```python
from build123d import *

# Parameters (mm, degrees)
BOSS_EXTRUDE1_DEPTH             = 3
CUT_EXTRUDE1_DEPTH              = 19.761966848
SKETCH3_W                       = 16.06
SKETCH3_H                       = 1.22
CUT_EXTRUDE2_DEPTH              = 3
CUT_EXTRUDE3_DEPTH              = 12.557681428
CUT_EXTRUDE3_DEPTH_BACK         = 12.557681428
SKETCH5_W                       = 1.3
SKETCH5_H                       = 3.6
CUT_EXTRUDE4_DEPTH              = 1.6
CUT_EXTRUDE5_DEPTH              = 1.6
SKETCH8_W                       = 0.3
SKETCH8_H                       = 1.3
BOSS_EXTRUDE3_DEPTH             = 0.3
CUT_EXTRUDE6_REACH              = 13.558
SKETCH9_W                       = 0.97
SKETCH9_H                       = 0.7
SKETCH10_W                      = 1.3
SKETCH10_H                      = 0.995055469
CUT_EXTRUDE7_DEPTH              = 0.3
SKETCH11_W                      = 1.3
SKETCH11_H                      = 1.339878891
CUT_EXTRUDE8_DEPTH              = 0.3
SKETCH12_W                      = 0.22
SKETCH12_H                      = 2.3
BOSS_EXTRUDE4_DEPTH             = 0.3
SZKIC1_W                        = 4.81
SZKIC1_H                        = 6.619114068
WYTNIJ_WYCI_GNI_CIE1_DEPTH      = 12.050452479
WYTNIJ_WYCI_GNI_CIE1_DEPTH_BACK = 12.050452479


with BuildPart() as part:
    # Sketch1 → Boss-Extrude1 (new body)
    with BuildSketch(Plane.XY):
        with BuildLine():
            Line((4.729085478, -2.65), (4.875, -2.504085478))
            Line((4.875, -2.504085478), (5.125, -2.504085478))
            Line((5.125, -2.504085478), (5.270914522, -2.65))
            Line((5.270914522, -2.65), (5.729085478, -2.65))
            Line((5.729085478, -2.65), (5.875, -2.504085478))
            Line((5.875, -2.504085478), (6.125, -2.504085478))
            Line((6.125, -2.504085478), (6.270914522, -2.65))
            Line((6.270914522, -2.65), (6.729085478, -2.65))
            Line((6.729085478, -2.65), (6.875, -2.504085478))
            Line((6.875, -2.504085478), (7.125, -2.504085478))
            Line((7.125, -2.504085478), (7.270914522, -2.65))
            Line((7.270914522, -2.65), (10.3, -2.65))
            Line((10.3, -2.65), (10.3, 1.65))
            Line((10.3, 1.65), (9.52, 1.65))
            Line((9.52, 1.65), (9.52, -1.49))
            ThreePointArc((9.52, -1.49), (9.26, -1.75), (9, -1.49))
            Line((9, -1.49), (9, 1.65))
            Line((9, 1.65), (8.03, 1.65))
            Line((8.03, 1.65), (8.03, 2.65))
            Line((8.03, 2.65), (-8.03, 2.65))
            Line((-8.03, 2.65), (-8.03, 1.65))
            Line((-8.03, 1.65), (-9, 1.65))
            Line((-9, 1.65), (-9, -1.49))
            ThreePointArc((-9, -1.49), (-9.26, -1.75), (-9.52, -1.49))
            Line((-9.52, -1.49), (-9.52, 1.65))
            Line((-9.52, 1.65), (-10.3, 1.65))
            Line((-10.3, 1.65), (-10.3, -2.65))
            Line((-10.3, -2.65), (-7.270914522, -2.65))
            Line((-7.270914522, -2.65), (-7.125, -2.504085478))
            Line((-7.125, -2.504085478), (-6.875, -2.504085478))
            Line((-6.875, -2.504085478), (-6.729085478, -2.65))
            Line((-6.729085478, -2.65), (-6.270914522, -2.65))
            Line((-6.270914522, -2.65), (-6.125, -2.504085478))
            Line((-6.125, -2.504085478), (-5.875, -2.504085478))
            Line((-5.875, -2.504085478), (-5.729085478, -2.65))
            Line((-5.729085478, -2.65), (-5.270914522, -2.65))
            Line((-5.270914522, -2.65), (-5.125, -2.504085478))
            Line((-5.125, -2.504085478), (-4.875, -2.504085478))
            Line((-4.875, -2.504085478), (-4.729085478, -2.65))
            Line((-4.729085478, -2.65), (-4.270914522, -2.65))
            Line((-4.270914522, -2.65), (-4.125, -2.504085478))
            Line((-4.125, -2.504085478), (-3.875, -2.504085478))
            Line((-3.875, -2.504085478), (-3.729085478, -2.65))
            Line((-3.729085478, -2.65), (-3.270914522, -2.65))
            Line((-3.270914522, -2.65), (-3.125, -2.504085478))
            Line((-3.125, -2.504085478), (-2.875, -2.504085478))
            Line((-2.875, -2.504085478), (-2.729085478, -2.65))
            Line((-2.729085478, -2.65), (-2.270914522, -2.65))
            Line((-2.270914522, -2.65), (-2.125, -2.504085478))
            Line((-2.125, -2.504085478), (-1.875, -2.504085478))
            Line((-1.875, -2.504085478), (-1.729085478, -2.65))
            Line((-1.729085478, -2.65), (-1.270914522, -2.65))
            Line((-1.270914522, -2.65), (-1.125, -2.504085478))
            Line((-1.125, -2.504085478), (-0.875, -2.504085478))
            Line((-0.875, -2.504085478), (-0.729085478, -2.65))
            Line((-0.729085478, -2.65), (-0.270914522, -2.65))
            Line((-0.270914522, -2.65), (-0.125, -2.504085478))
            Line((-0.125, -2.504085478), (0.125, -2.504085478))
            Line((0.125, -2.504085478), (0.270914522, -2.65))
            Line((0.270914522, -2.65), (0.729085478, -2.65))
            Line((0.729085478, -2.65), (0.875, -2.504085478))
            Line((0.875, -2.504085478), (1.125, -2.504085478))
            Line((1.125, -2.504085478), (1.270914522, -2.65))
            Line((1.270914522, -2.65), (1.729085478, -2.65))
            Line((1.729085478, -2.65), (1.875, -2.504085478))
            Line((1.875, -2.504085478), (2.125, -2.504085478))
            Line((2.125, -2.504085478), (2.270914522, -2.65))
            Line((2.270914522, -2.65), (2.729085478, -2.65))
            Line((2.729085478, -2.65), (2.875, -2.504085478))
            Line((2.875, -2.504085478), (3.125, -2.504085478))
            Line((3.125, -2.504085478), (3.270914522, -2.65))
            Line((3.270914522, -2.65), (3.729085478, -2.65))
            Line((3.729085478, -2.65), (3.875, -2.504085478))
            Line((3.875, -2.504085478), (4.125, -2.504085478))
            Line((4.125, -2.504085478), (4.270914522, -2.65))
            Line((4.270914522, -2.65), (4.729085478, -2.65))
        make_face()
    extrude(amount=BOSS_EXTRUDE1_DEPTH)

    # Sketch2 → Cut-Extrude1 (cut, through all)
    with BuildSketch(Plane(origin=(8.03, 0, 0), x_dir=(0, 0, -1), z_dir=(1, 0, 0))):
        Polygon((-2.4, 2.65), (-2.32, 1.65), (0.208388731, 1.65), (0.247686287, 2.908353898), align=None)
    extrude(amount=-CUT_EXTRUDE1_DEPTH, mode=Mode.SUBTRACT)

    # Sketch3 → Cut-Extrude2 (cut)
    with BuildSketch(Plane(origin=(0, 1.65, 0), x_dir=(1, 0, 0), z_dir=(0, 1, 0))):
        with Locations((0, -1.61)):
            Rectangle(SKETCH3_W, SKETCH3_H)
    extrude(amount=-CUT_EXTRUDE2_DEPTH, mode=Mode.SUBTRACT)

    # Sketch4 → Cut-Extrude3 (cut, two sides)
    with BuildSketch(Plane(origin=(0, 1.65, 0), x_dir=(1, 0, 0), z_dir=(0, 1, 0))) as cut_extrude3_sk:
        Polygon((7.12, -1), (7.12, -0.61), (6.87, -0.61), (6.87, -1.06), (7.12, -1.06), align=None)
    extrude(amount=CUT_EXTRUDE3_DEPTH, mode=Mode.SUBTRACT)
    extrude(cut_extrude3_sk.sketch, amount=-CUT_EXTRUDE3_DEPTH_BACK, mode=Mode.SUBTRACT)

    # Sketch5 → Cut-Extrude4 (cut)
    with BuildSketch(Plane.ZY.offset(10.3)):
        with Locations((1.5, -0.85)):
            Rectangle(SKETCH5_W, SKETCH5_H)
    extrude(amount=-CUT_EXTRUDE4_DEPTH, mode=Mode.SUBTRACT)

    # Sketch6 → Cut-Extrude5 (cut)
    with BuildSketch(Plane(origin=(10.3, 0, 0), x_dir=(0, 0, -1), z_dir=(1, 0, 0))):
        Polygon((-2.15, 0.95), (-0.85, 0.95), (-0.85, -1.49), (-0.85, -2.65), (-2.15, -2.65), (-2.15, -1.49), align=None)
    extrude(amount=-CUT_EXTRUDE5_DEPTH, mode=Mode.SUBTRACT)

    # Sketch8 → Boss-Extrude3 (add)
    with BuildSketch(Plane.ZY.offset(8.7)):
        with Locations((2, -2)):
            Rectangle(SKETCH8_W, SKETCH8_H)
    boss_extrude3 = extrude(amount=BOSS_EXTRUDE3_DEPTH)

    # Cut-Extrude6: up to this face of the body (flat: up to its plane)
    cut_extrude6_end = Plane(part.part.faces().sort_by_distance((-0.005359277, -1.35, 1.610444372))[0])
    # Sketch9 → Cut-Extrude6 (cut, up to the picked face)
    with BuildSketch(Plane(origin=(0, 1.65, 0), x_dir=(1, 0, 0), z_dir=(0, 1, 0)), mode=Mode.PRIVATE) as cut_extrude6_sk1:
        with Locations((-8.515, -1.61)):
            Rectangle(SKETCH9_W, SKETCH9_H)
    cut_extrude6_tool1 = split(extrude(cut_extrude6_sk1.sketch, amount=-CUT_EXTRUDE6_REACH, mode=Mode.PRIVATE), bisect_by=cut_extrude6_end, keep=Keep.BOTH, mode=Mode.PRIVATE)
    cut_extrude6 = cut_extrude6_tool1.solids().sort_by(Axis((-8.515, 1.65, 1.61), (0, -1, 0)))[0]
    add(cut_extrude6, mode=Mode.SUBTRACT)

    # Mirror2: Cut-Extrude6 across plane
    add(cut_extrude6.mirror(Plane.ZY), mode=Mode.SUBTRACT)

    # Sketch10 → Cut-Extrude7 (cut)
    with BuildSketch(Plane.ZY.offset(9)):
        with Locations((1.5, 1.447527735)):
            Rectangle(SKETCH10_W, SKETCH10_H)
    extrude(amount=-CUT_EXTRUDE7_DEPTH, mode=Mode.SUBTRACT)

    # Sketch11 → Cut-Extrude8 (cut)
    with BuildSketch(Plane(origin=(9, 0, 0), x_dir=(0, 0, -1), z_dir=(1, 0, 0))):
        with Locations((-1.5, 1.619939446)):
            Rectangle(SKETCH11_W, SKETCH11_H)
    extrude(amount=-CUT_EXTRUDE8_DEPTH, mode=Mode.SUBTRACT)

    # Sketch12 → Boss-Extrude4 (add)
    with BuildSketch(Plane.ZY.offset(8.7)):
        with Locations((0.96, 0.5)):
            Rectangle(SKETCH12_W, SKETCH12_H)
    boss_extrude4 = extrude(amount=BOSS_EXTRUDE4_DEPTH)

    # Mirror4: Boss-Extrude4 across plane
    add(boss_extrude4.mirror(Plane.ZY))

    # Mirror5: Boss-Extrude3 across plane
    add(boss_extrude3.mirror(Plane.ZY))

    # Szkic1 → Wytnij-wyciągnięcie1 (cut, two sides)
    with BuildSketch(Plane.XY.offset(3)) as wytnij_wyci_gni_cie1_sk:
        with Locations((0, -0.145396272)):
            Rectangle(SZKIC1_W, SZKIC1_H)
    extrude(amount=WYTNIJ_WYCI_GNI_CIE1_DEPTH, mode=Mode.SUBTRACT)
    extrude(wytnij_wyci_gni_cie1_sk.sketch, amount=-WYTNIJ_WYCI_GNI_CIE1_DEPTH_BACK, mode=Mode.SUBTRACT)


with BuildPart() as wytnij_wyci_gni_cie1_piece_1:
    # of the separate pieces the step leaves, piece 1, a body of its own (wytnij_wyci_gni_cie1_pieces)
    add(part.part.solids().sort_by_distance((-2.405, -2.65, 0))[0])


with BuildPart() as wytnij_wyci_gni_cie1_piece_2:
    # of the separate pieces the step leaves, piece 2, a body of its own (wytnij_wyci_gni_cie1_pieces)
    add(part.part.solids().sort_by_distance((3.729085478, -2.65, 0))[0])


with BuildPart() as wytnij_wyci_gni_cie1_piece_1_1:
    # Obiekt-Przenieś/Kopiuj1: moved
    add(wytnij_wyci_gni_cie1_piece_1.part.moved(Location((4.81, 0, 0))))

    # Połącz1: union Wytnij-wyciągnięcie1 piece 2
    add(wytnij_wyci_gni_cie1_piece_2.part)


solid = wytnij_wyci_gni_cie1_piece_1_1.part
```
Can you work these out from the model? Positions are in its coordinate system, mm. A direction names the side the tool comes from. Round coordinates to 2 decimals unless told otherwise and drop trailing zeros. Order: outer loops, then holes, each group sorted by start corner. A loop starts at its lowest first (then second) coordinate and runs counter-clockwise, first axis right, second up.
(1) If I drill on L1, parallel to X at y = 0.5, z = 2.4; L2, parallel to Z at x = 1.5, y = 1.1; L3, parallel to X at y = 1.2, z = 1.9, over which ranges is the centre line in solid material (lowest first)?
Results are:
L1: x = -5.49 to -4.71, -4.19 to 9, 9.52 to 10.3
L2: z = 0 to 1, 2.22 to 3
L3: x = -5.49 to -4.71, 9.52 to 10.3
(2) If we section it at B-B (x = -3.5): Please give me the cut outline in (y, z), plus the area to 3 significant figures.
Results are:
outline: (-2.65, 0) - (1.65, 0) - (1.65, 1.26) - (-1.35, 1.26) - (-1.35, 1.96) - (1.65, 1.96) - (1.65, 3) - (-2.65, 3) - close
area: 10.8 mm2
(3) If we section it at A-A (x = 9.26): Please give me the cut outline in (y, z), plus the area to 3 significant figures.
Results are:
outline: (-2.65, 0) - (-1.75, 0) - (-1.75, 0.85) - (-2.65, 0.85) - close; (-2.65, 2.15) - (-1.75, 2.15) - (-1.75, 3) - (-2.65, 3) - close
area: 1.53 mm2
(4) We'd pull the mould along X, two halves only. Please class faces 1 (the face through (-5.49, 0, 0.5)), 2 (the face through (2.3, 1.65, 0.5)), 3 (the face through (9.52, 1.1, 1.5)): +X half, -X half, draft (parallel to the pull), parting line (faces both ways), or undercut.
Results are:
face 1: -X half
face 2: draft
face 3: undercut
(5) On a 3-axis mill with a long thin cutter (end or side, diameter ignored), from which of +Z, -Z, +X, -X, +Y, -Y can I reach the whole of each face in a straight line? I mean faces 4 (the face through (-5, -1, 2.15)), 5 (the face through (7.6, 0.2, 1)), 6 (the face through (-4.19, 0.1, 0.5)). Say none if no direction works.
Results are:
face 4: -X, -Y
face 5: +Y
face 6: +Z, -Z, +Y
(6) If we section it at C-C (y = -0.2): Count the separate pieces of the cut face and the enclosed holes in it, plus the area to 3 significant figures.
Results are:
separate pieces: 6
enclosed holes: 0
area: 26.8 mm2
(7) I'm going to push a flat-ended pin straight in: pin 1 (1.5 mm diameter, centred on x = 2.5, y = 0.5, fed in from -Z). Where does the tip first touch, or does it pass through?
Results are:
pin 1: stops at z = 0
